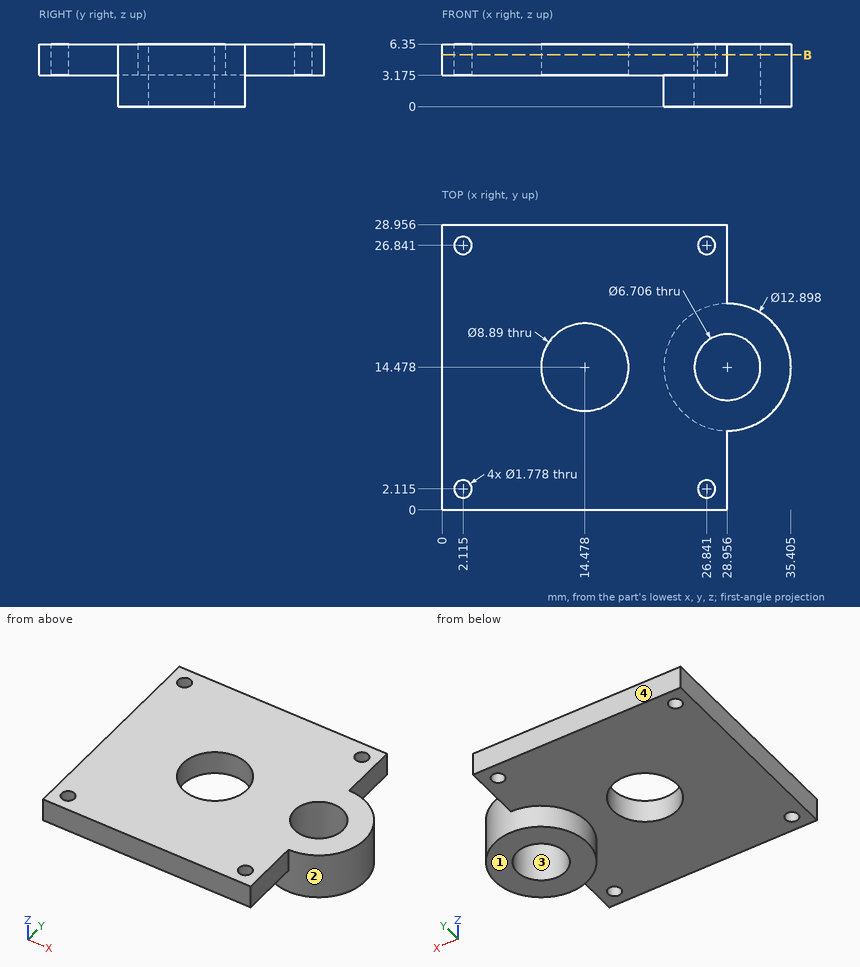
The figure shows three views and two pictorial views of one solid part (mm, origin at its lowest corner). Answer the questions. Give positions to 0.01 mm unless a question says otherwise; leave off trailing zeros. Write each question's results on one line, items separated by ' | '.
Q1. Consider L1, parallel to Y at x = 30, z = 2 (1 decimal); L2, parallel to Y at x = 17, z = 4.75 (1 decimal); L3, parallel to X at y = 12.75, z = 4.5 (1 decimal). Determine where each line is inside the solid, lowest interval first. Write a range as from..to.
Output values:
L1: 8.1..11.3, 17.7..20.8 | L2: 0..10.8, 18.1..29 | L3: 0..10.4, 18.6..26.1, 31.8..35.2
Q2. For a pull along Y with two mould halves and no side action, classify the marked faces 1, 2, 3 and 4 as released by +Y, released by -Y, zero draft, split by the parting line, or undercut.
Output values:
face 1: zero draft | face 2: split by the parting line | face 3: undercut | face 4: released by +Y
Q3. Section B-B, the plane z = 5.25 is taken. Count the separate pieces of the cut face and the enclosed holes in it.
Output values:
separate pieces: 1 | enclosed holes: 6
Q4. Flat-ended cylindrical pins translate along their axes: P1, Ø1, axis at y = 19.5, z = 4.5, coming from the +X side (1 decimal); P2, Ø8.5, axis at x = 14, y = 18, coming from the -Z side (3 decimals); P3, Ø1.6, axis at y = 3.5, z = 5, coming from the +X side. Find the tip coordinate at first contact, or state that the pin passes through.
Output values:
P1: x = 33.6 | P2: z = 3.175 | P3: x = 28.96
